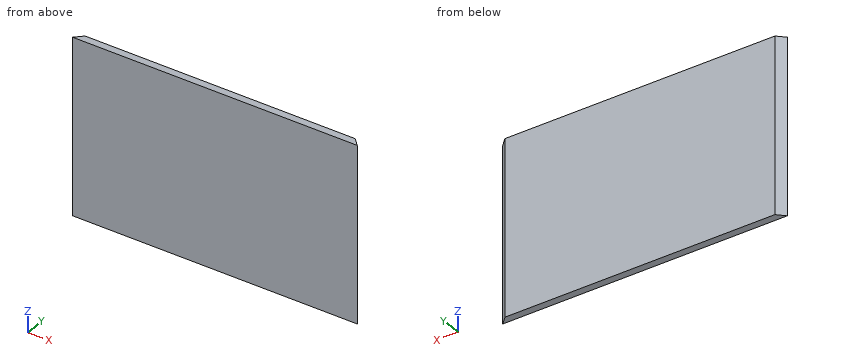
```python
from build123d import *

# Parameters (mm, degrees)
SKETCH2_W           = 254
SKETCH2_H           = 152.4
BOSS_EXTRUDE1_DEPTH = 3.175
CHAMFER1_SIZE       = 10
CHAMFER2_SIZE       = 10


with BuildPart() as part:
    # Sketch2 → Boss-Extrude1 (new, symmetric)
    with BuildSketch(Plane(origin=(0, 0, 0), x_dir=(1, 0, 0), z_dir=(0, 1, 0))):
        Rectangle(SKETCH2_W, SKETCH2_H)
    extrude(amount=BOSS_EXTRUDE1_DEPTH, both=True)

    # Chamfer1
    # the kernel refuses this chamfer: 10 mm, written as the material it takes off along each edge
    with BuildSketch(Plane(origin=(-127, 3.175, -101.91682988), x_dir=(-0.027495876610586317, -0.9996219169112968, 0), z_dir=(0, 0, 1))) as chamfer1_piece_1:
        Polygon((CHAMFER1_SIZE * 0.999621916911, CHAMFER1_SIZE * 0.0274958766106), (-CHAMFER1_SIZE * 0.0274958766106, CHAMFER1_SIZE * 0.999621916911), (0, 0), align=None)
    extrude(amount=203.833659759, mode=Mode.SUBTRACT)

    # Chamfer2
    # the kernel refuses this chamfer: 10 mm, written as the material it takes off along each edge
    with BuildSketch(Plane(origin=(127, 3.175, 101.91682988), x_dir=(-0.9996219169112968, 0.02749587661058636, 0), z_dir=(0, 0, -1))) as chamfer2_piece_1:
        Polygon((CHAMFER2_SIZE * 0.999621916911, -CHAMFER2_SIZE * 0.0274958766106), (-CHAMFER2_SIZE * 0.0274958766106, -CHAMFER2_SIZE * 0.999621916911), (0, 0), align=None)
    extrude(amount=203.833659759, mode=Mode.SUBTRACT)


solid = part.part
```
Input: part model. Units: mm. Frame: model coordinates. Coordinates: 2 decimals unless noted, no trailing zeros. Loops run counter-clockwise (first coordinate to the right, second up) from the corner with the lowest first, then second, coordinate; pieces in that order, holes last. Notation, with made-up numbers: M 62,-27.5 L 86,-27.5 A31 cw 86,-0.5 Z; hole C 50.5,76.25 d3. An arc over 180 degrees is marked long. Use a Markdown table: item, result. Add a question column.
1) Section A-A, the plane z = -16. Return the cut outline in (x, y) (3 decimals), plus the area to 3 significant figures.
2) Line query: L1, parallel to X at y = -2.5, z = 49 (3 decimals); L2, parallel to X at y = 1.5, z = 57.5 (3 decimals). Output: solid intervals per line, ascending. Write a range as from..to.
3) Section B-B, the plane y = -0.25. Return the cut outline in (x, z) (3 decimals).
4) Pin query (flat end, axial travel): P1, Ø3, axis at y = 2.5, z = -20.5, coming from the -X side (3 decimals); P2, Ø1.5, axis at y = -1.5, z = -57, coming from the -X side (3 decimals). Return the tip coordinate at first contact, or that it passes through.
Answer below:
| question | item | result |
|---|---|---|
| 1 | outline | M -123.35,-3.175 L 123.35,-3.175 L 117,3.175 L -117,3.175 Z |
| 1 | area | 1,530 mm2 |
| 2 | L1 | -122.675..122.675 |
| 2 | L2 | -118.675..118.675 |
| 3 | outline | M -120.425,-76.2 L 120.425,-76.2 L 120.425,76.2 L -120.425,76.2 Z |
| 4 | P1 | x = -119.175 |
| 4 | P2 | x = -122.425 |
